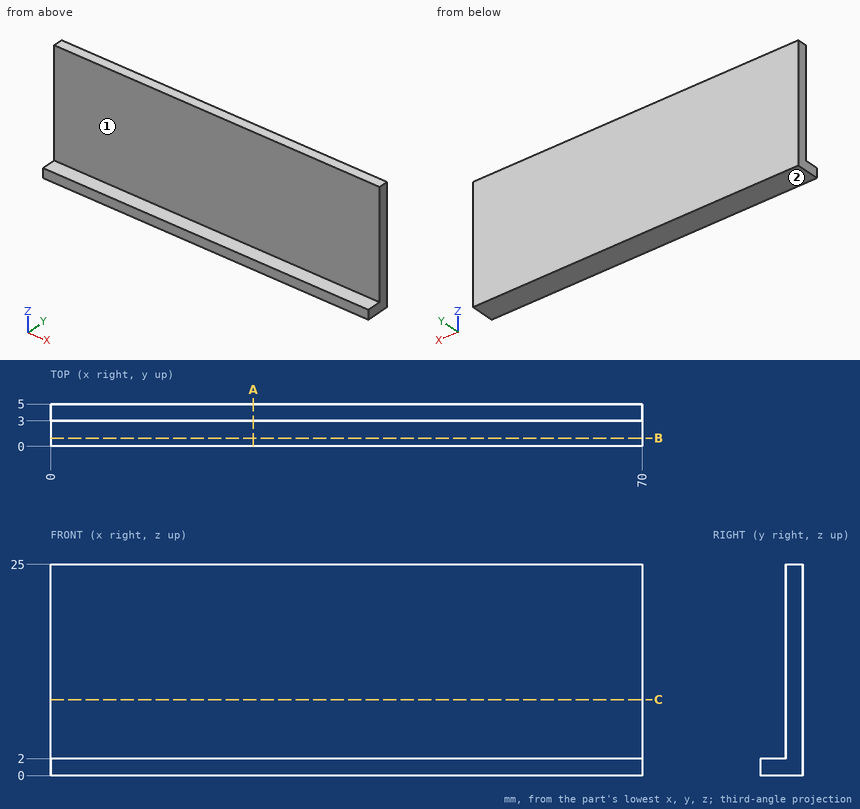
The figure shows three views and two pictorial views of one solid part (mm, origin at its lowest corner). Answer the questions. A direction names the side the tool comes from. Round coordinates to 2 decimals unless told otherwise and drop trailing zeros. Write each loop counter-clockwise with the first axis right and the second up, starting at its lowest first coordinate (ties: lowest second). Pieces come first, ordered by that corner, then holes. Notation, with made-up numbers: M 80.5,71.5 L 128.5,71.5 A30 cw 128.5,104.5 Z; hole C -19.75,58.25 d2. An arc over 180 degrees is marked long. Use a Markdown table: item, result.
1) The part is cut by section A-A on x = 24. Give the vertices of the cut face in (y, z).
Taken from the geometry:
| item | result |
|---|---|
| outline | M 0,0 L 5,0 L 5,25 L 3,25 L 3,2 L 0,2 Z |
2) The part is cut by section B-B on y = 0.95. Give the vertices of the cut face in (x, z), plus the area to 3 significant figures.
Taken from the geometry:
| item | result |
|---|---|
| outline | M 0,0 L 70,0 L 70,2 L 0,2 Z |
| area | 140 mm2 |
3) The part is cut by section C-C on z = 9. Give the vertices of the cut face in (x, y).
Taken from the geometry:
| item | result |
|---|---|
| outline | M 0,3 L 70,3 L 70,5 L 0,5 Z |
4) Consider line 1 (Y direction, x = 19, z = 19.25); line 2 (Z direction, x = 13, y = 1.15). Determine where each line is inside the solid, lowest interval first. Write a range as [from, to].
Taken from the geometry:
| item | result |
|---|---|
| line 1 | y = [3, 5] |
| line 2 | z = [0, 2] |
5) Flat-ended cylindrical pins translate along their axes: pin 1 (0.9 mm diameter, centred on x = 32.5, y = 1, fed in from +Z); pin 2 (1.5 mm diameter, centred on x = 29.5, z = 6.5, fed in from -Y). Find the tip coordinate at first contact, or state that the pin passes through.
Taken from the geometry:
| item | result |
|---|---|
| pin 1 | stops at z = 2 |
| pin 2 | stops at y = 3 |
6) Which of the six approach directions +Z, -Z, +X, -X, +Y, -Y give full straight-line access (tool end or side, diameter ignored) to the marked faces 1 and 2?
Taken from the geometry:
| item | result |
|---|---|
| face 1 | +Z, +X, -X, -Y |
| face 2 | -Z, +X, -X, +Y, -Y |
